For this review, take the finished solid that the model builds, in its own axes (mm). Face numbers are marked on the shaded views. Coordinates: 2 decimals unless noted, no trailing zeros. Write each loop counter-clockwise with the first axis right and the second up, starting at its lowest first coordinate (ties: lowest second). Pieces come first, ordered by that corner, then holes.
```python
from build123d import *

# Parameters (mm, degrees)
BOSS_EXTRUDE1_DEPTH = 1.5
SKETCH4_W           = 2
SKETCH4_H           = 7.019019915
CUT_EXTRUDE2_DEPTH  = 3


with BuildPart() as part:
    # Sketch2 → Boss-Extrude1 (new, symmetric)
    with BuildSketch(Plane.XY):
        with BuildLine():
            Line((294.5, -67.353443934), (299.5, -67.353443934))
            Line((299.5, -67.353443934), (299.5, -65.649534053))
            ThreePointArc((299.5, -65.649534053), (182.278534334, -18.599191723), (57.25, -0.641677179))
            Line((57.25, -0.641677179), (57.25, -4.102198064))
            Line((57.25, -4.102198064), (51.25, -4.102198064))
            ThreePointArc((51.25, -4.102198064), (50.542893219, -4.395091282), (50.25, -5.102198064))
            Line((50.25, -5.102198064), (50.25, -34.102198064))
            Line((50.25, -34.102198064), (57.25, -34.102198064))
            Line((57.25, -34.102198064), (57.25, -37.402198064))
            Line((57.25, -37.402198064), (50.25, -37.402198064))
            Line((50.25, -37.402198064), (50.25, -44.402198064))
            Line((50.25, -44.402198064), (57.25, -44.402198064))
            Line((57.25, -44.402198064), (57.25, -47.402198064))
            Line((57.25, -47.402198064), (50.25, -47.402198064))
            Line((50.25, -47.402198064), (50.25, -53.402198064))
            Line((50.25, -53.402198064), (67.25, -53.402198064))
            Line((67.25, -53.402198064), (67.25, -38.8))
            Line((67.25, -38.8), (67.25, -21.521364961))
            ThreePointArc((67.25, -21.521364961), (70.406305806, -14.230010507), (77.882769957, -11.541404932))
            ThreePointArc((77.882769957, -11.541404932), (101.0737918, -13.534149792), (124.152314439, -16.563393762))
            ThreePointArc((124.152314439, -16.563393762), (124.759050209, -16.900693759), (125, -17.551725847))
            Line((125, -17.551725847), (125, -18.257285386))
            ThreePointArc((125, -18.257285386), (125.292893219, -18.964392167), (126, -19.257285386))
            Line((126, -19.257285386), (140, -19.257285386))
            Line((140, -19.257285386), (140, -22.257285386))
            Line((140, -22.257285386), (125, -22.257285386))
            Line((125, -22.257285386), (125, -26.257285386))
            Line((125, -26.257285386), (171.998789441, -26.257285386))
            ThreePointArc((171.998789441, -26.257285386), (217.028547909, -39.800007252), (260.649793668, -57.357666027))
            ThreePointArc((260.649793668, -57.357666027), (264.911240595, -61.04755196), (266.5, -66.455974249))
            Line((266.5, -66.455974249), (266.5, -84.321193081))
            ThreePointArc((266.5, -84.321193081), (267.378679656, -86.442513425), (269.5, -87.321193081))
            Line((269.5, -87.321193081), (273.5, -87.321193081))
            ThreePointArc((273.5, -87.321193081), (275.621320344, -86.442513425), (276.5, -84.321193081))
            Line((276.5, -84.321193081), (276.5, -69.703443934))
            Line((276.5, -69.703443934), (292.5, -69.703443934))
            ThreePointArc((292.5, -69.703443934), (293.207106781, -69.410550715), (293.5, -68.703443934))
            Line((293.5, -68.703443934), (293.5, -68.353443934))
            ThreePointArc((293.5, -68.353443934), (293.792893219, -67.646337153), (294.5, -67.353443934))
        make_face()
    extrude(amount=BOSS_EXTRUDE1_DEPTH, both=True)

    # Sketch4 → Cut-Extrude2 (cut)
    with BuildSketch(Plane.XY.offset(-1.5)):
        with Locations((298.5, -66.105228371)):
            Rectangle(SKETCH4_W, SKETCH4_H)
    extrude(amount=CUT_EXTRUDE2_DEPTH, mode=Mode.SUBTRACT)


solid = part.part
```
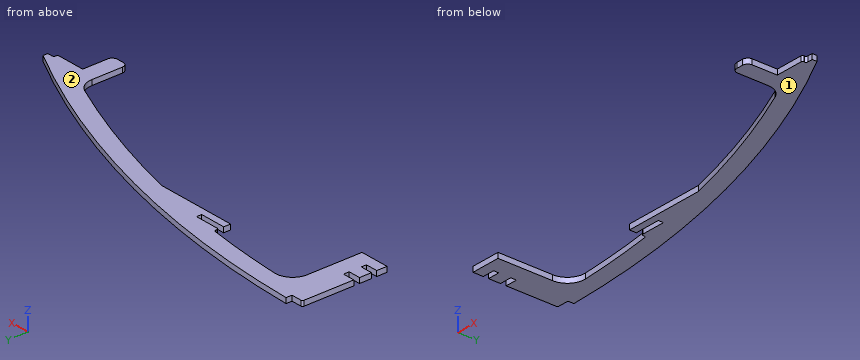
Q1. Add section B-B (y = -51). State the section outline as (x, z) points, then the cut area to 3 significant figures.
Ans:
outline: (50.25, -1.5) - (67.25, -1.5) - (67.25, 1.5) - (50.25, 1.5) - close; (246.13, -1.5) - (270.71, -1.5) - (270.71, 1.5) - (246.13, 1.5) - close
area: 125 mm2
Q2. Clearance check with flat-ended pins moving along their axes: pin 1 Ø1.5 at (x, y) = (182.5, -30) entering from -Z; pin 2 Ø0.9 at (x, z) = (55.5, -0.5) entering from +Y; pin 3 Ø1.5 at (y, z) = (-75.5, -0.5) entering from +X. State where each tip first meets the part, or that it passes through.
Ans:
pin 1: passes through
pin 2: stops at y = -4.1
pin 3: stops at x = 276.5
Q3. For probe 1 along X at (y, z) = (-47.5, 0.15); probe 2 along X at (y, z) = (-83, -0.35); probe 3 along Y at (x, z) = (258.5, 0.4), list the stretches that pass through material, from the lowest coordinate up.
Ans:
probe 1: x = 50.25 to 67.25, 237.58 to 263.13
probe 2: x = 266.5 to 276.5
probe 3: y = -56.38 to -45.44
Q4. Add section C-C (y = -80). State the section outline as (x, z) points, then the cut area to 3 significant figures.
Ans:
outline: (266.5, -1.5) - (276.5, -1.5) - (276.5, 1.5) - (266.5, 1.5) - close
area: 30.0 mm2
Q5. Draft analysis for pull direction Z (two halves, no side actions). For the marked faces 1 and 2, state which applies: +Z half, -Z half, draft (parallel to the pull), parting line (faces both ways), or undercut.
Ans:
face 1: -Z half
face 2: +Z half
Q6. Add section A-A (x = 136.5). State the section outline as (y, z) points, then the cut area to 3 significant figures.
Ans:
outline: (-26.26, -1.5) - (-22.26, -1.5) - (-22.26, 1.5) - (-26.26, 1.5) - close; (-19.26, -1.5) - (-8.46, -1.5) - (-8.46, 1.5) - (-19.26, 1.5) - close
area: 44.4 mm2
Q7. Add section D-D (x = 203). State the section outline as (y, z) points.
Ans:
outline: (-35.1, -1.5) - (-24.61, -1.5) - (-24.61, 1.5) - (-35.1, 1.5) - close
